Design review of the part built by this model. Coordinates are the model's own, in mm. A direction names the side the tool comes from. Give positions to 0.01 mm unless a question says otherwise; leave off trailing zeros. Loops run counter-clockwise (first coordinate to the right, second up) from the corner with the lowest first, then second, coordinate; pieces in that order, holes last. Notation, with made-up numbers: (9, 0) -> (16, 0) arc R26 ccw to (16, 17) -> close; hole circle Ø1 at (24, 69.5). An arc over 180 degrees is marked (long way). Use CSV: the item, a comma, the result in double quotes. Start each with the question number.
Item 1: We need section D-D (x = 14.5). State the section outline as (y, z) points.
Item 2: We need section B-B (y = 21). State the section outline as (x, z) points.
Item 3: For faces 4 (the face through (47.5, 21.7, 0)), 5 (the face through (45.4, 4, 2.5)), 6 (the face through (41.6, 2.03, 0.57)), list the 3-axis set-ups (+Z, -Z, +X, -X, +Y, -Y) from which the entire face can be reached by the end or side of a thin tool; tool diameter is ignored.
Item 4: Wall thickness on line 1 along X through (y, z) = (1.55, 2.5); line 2 along X through (y, z) = (32, 3.75); line 3 along Y through (x, z) = (33.5, -1.25): over which ranges is each line inside the solid? List them lowest first. Write a range as from..to.
Item 5: We need section A-A (x = 25.5). State the section outline as (y, z) points.
Item 6: The part is to be moulded in two halves that separate along Y. For faces 1 (the face through (47, 20, 3)), 2 (the face through (5, 0, 2)), 3 (the face through (6.036, 2.028, 2.175)), say which applies: +Y half, -Y half, draft (parallel to the pull), parting line (faces both ways), or undercut.
Item 7: We need section C-C (x = 34). State the section outline as (y, z) points.
Item 8: Clearance check with flat-ended pins moving along their axes: pin 1 (10.5 mm diameter, centred on x = 6.5, y = 11.5, fed in from +Z); pin 2 (8.5 mm diameter, centred on x = 28, z = -1.5, fed in from -Y); pin 3 (14.5 mm diameter, centred on x = 41.5, y = 15, fed in from -Z). State where each tip first meets the part, or that it passes through.
from build123d import *

# Parameters (mm, degrees)
SKETCH_1_W           = 10
SKETCH_1_H           = 5
EXTRUDE_1_DEPTH      = 4
SKETCH_3_R           = 1.5
CUT_EXTRUDE_1_DEPTH  = 4
SKETCH_4_W           = 4
SKETCH_4_H           = 5
EXTRUDE_2_DEPTH      = 40
SKETCH_5_W           = 5
SKETCH_5_H           = 4
EXTRUDE_3_DEPTH      = 47
SKETCH_7_W           = 4
SKETCH_7_H           = 5
EXTRUDE_4_DEPTH      = 40
SKETCH_8_W           = 5
SKETCH_8_H           = 4
EXTRUDE_5_DEPTH      = 6
SKETCH_10_R          = 1.5
CUT_EXTRUDE_2_DEPTH  = 6
EXTRUDE_6_DEPTH      = 6
EXTRUDE_6_DEPTH_BACK = 11
SKETCH_11_W          = 15
SKETCH_11_H          = 4
FILLET_1_R           = 5
SKETCH_12_R          = 2
CUT_EXTRUDE_3_DEPTH  = 6
FILLET_2_R           = 5
FILLET_3_R           = 5
FILLET_4_R           = 2
FILLET_5_R           = 2


with BuildPart() as part:
    # 草图1 → 凸台-拉伸1 (new body)
    with BuildSketch(Plane(origin=(0, 0, 0), x_dir=(1, 0, 0), z_dir=(0, 1, 0))):
        with Locations((5, -2.5)):
            Rectangle(SKETCH_1_W, SKETCH_1_H)
    extrude(amount=EXTRUDE_1_DEPTH)

    # 草图3 → 切除-拉伸1 (cut)
    with BuildSketch(Plane(origin=(0, 4, 0), x_dir=(1, 0, 0), z_dir=(0, 1, 0))):
        with Locations(Location((7.5, -2.5, 0), (0, 0, 270))):
            Circle(SKETCH_3_R)
    extrude(amount=-CUT_EXTRUDE_1_DEPTH, mode=Mode.SUBTRACT)

    # 草图4 → 凸台-拉伸2 (add)
    with BuildSketch(Plane(origin=(0, 4, 0), x_dir=(1, 0, 0), z_dir=(0, 1, 0))):
        with Locations((2, -2.5)):
            Rectangle(SKETCH_4_W, SKETCH_4_H)
    extrude(amount=EXTRUDE_2_DEPTH)

    # 草图5 → 凸台-拉伸3 (add)
    with BuildSketch(Plane(origin=(4, 0, 0), x_dir=(0, 0, -1), z_dir=(1, 0, 0))):
        with Locations((-2.5, 42)):
            Rectangle(SKETCH_5_W, SKETCH_5_H)
    extrude(amount=EXTRUDE_3_DEPTH)

    # 草图7 → 凸台-拉伸4 (add)
    with BuildSketch(Plane(origin=(0, 40, 0), x_dir=(-1, 0, 0), z_dir=(0, -1, 0))):
        with Locations((-49, -2.5)):
            Rectangle(SKETCH_7_W, SKETCH_7_H)
    extrude(amount=EXTRUDE_4_DEPTH)

    # 草图8 → 凸台-拉伸5 (add)
    with BuildSketch(Plane.ZY.offset(-47)):
        with Locations((2.5, 2)):
            Rectangle(SKETCH_8_W, SKETCH_8_H)
    extrude(amount=EXTRUDE_5_DEPTH)

    # 草图10 → 切除-拉伸2 (cut)
    with BuildSketch(Plane(origin=(0, 0, 0), x_dir=(-1, 0, 0), z_dir=(0, -1, 0))):
        with Locations(Location((-43.5, -2.5, 0), (0, 0, 90))):
            Circle(SKETCH_10_R)
    extrude(amount=-CUT_EXTRUDE_2_DEPTH, mode=Mode.SUBTRACT)

    # 草图11 → 凸台-拉伸6 (add, two sides: drawn at the far end of the back side and taken through both)
    with BuildSketch(Plane(origin=(0, 0, 0), x_dir=(-1, 0, 0), z_dir=(0, 0, -1)).offset(-EXTRUDE_6_DEPTH_BACK)):
        with Locations((-25.5, 42)):
            Rectangle(SKETCH_11_W, SKETCH_11_H)
    extrude(amount=EXTRUDE_6_DEPTH + EXTRUDE_6_DEPTH_BACK)

    # 圆角1
    fillet_1_edges = [part.edges().sort_by_distance(p)[0] for p in [
        (33, 42, 5),
        (33, 42, 0),
        (18, 42, 5),
        (18, 42, 0),
    ]]
    fillet(fillet_1_edges, radius=FILLET_1_R)

    # 草图12 → 切除-拉伸3 (cut)
    with BuildSketch(Plane(origin=(0, 44, 0), x_dir=(1, 0, 0), z_dir=(0, 1, 0))):
        with Locations(Location((25.5, -2.5, 0), (0, 0, 270))):
            Circle(SKETCH_12_R)
    extrude(amount=-CUT_EXTRUDE_3_DEPTH, mode=Mode.SUBTRACT)

    # 圆角2
    fillet_2_edges = [part.edges().sort_by_distance(p)[0] for p in [
        (18, 42, -6),
        (33, 42, -6),
        (33, 42, 11),
        (18, 42, 11),
    ]]
    fillet(fillet_2_edges, radius=FILLET_2_R)

    # 圆角3
    fillet_3_edges = [part.edges().sort_by_distance(p)[0] for p in [
        (4, 40, 2.5),
        (47, 40, 2.5),
    ]]
    fillet(fillet_3_edges, radius=FILLET_3_R)

    # 圆角4
    fillet_4_edges = [part.edges().sort_by_distance(p)[0] for p in [
        (10, 2, 0),
        (10, 2, 5),
    ]]
    fillet(fillet_4_edges, radius=FILLET_4_R)

    # 圆角5
    fillet_5_edges = [part.edges().sort_by_distance(p)[0] for p in [
        (0, 44, 2.5),
        (51, 44, 2.5),
        (41, 2, 0),
        (41, 2, 5),
    ]]
    fillet(fillet_5_edges, radius=FILLET_5_R)


solid = part.part
Results found:
1,outline,"(40, -0.23) -> (44, -0.23) -> (44, 5.23) -> (40, 5.23) -> close"
2,outline,"(0, 0) -> (4, 0) -> (4, 5) -> (0, 5) -> close; (47, 0) -> (51, 0) -> (51, 5) -> (47, 5) -> close"
3,face 4,"-Z, +X, +Y, -Y"
3,face 5,"+Z, -Z"
3,face 6,"-Z, -Y"
4,line 1,"0..6, 9..10, 41..42, 45..51"
4,line 2,"0..4, 47..51"
4,line 3,"40..44"
5,outline,"(40, -6) -> (44, -6) -> (44, 0.5) -> (40, 0.5) -> close; (40, 4.5) -> (44, 4.5) -> (44, 11) -> (40, 11) -> close"
6,face 1,"undercut"
6,face 2,"-Y half"
6,face 3,"draft"
7,outline,"(40, -2) -> (44, -2) -> (44, 7) -> (40, 7) -> close"
8,pin 1,"z = 5"
8,pin 2,"y = 40"
8,pin 3,"z = 0"
